Check sheet for the modelled part. Datum: model origin and axes. Units: mm. Give positions to 0.01 mm unless a question says otherwise; leave off trailing zeros. Loops run counter-clockwise (first coordinate to the right, second up) from the corner with the lowest first, then second, coordinate; pieces in that order, holes last. Notation, with made-up numbers: (15, 72.5) - (70, 72.5) arc R7 cw to (70, 81.5) - close; hole circle Ø7 at (-18, -29). An arc over 180 degrees is marked (long way). Answer in a Markdown table with one row per item. Add a question column.
(1) Draft check along Z on faces 1 (the face through (-2.44, 0.69, -0.54)), 2 (the face through (-1.22, -0.69, -0.27)). Enter one of: released by +Z, released by -Z, zero draft, split by the parting line, or undercut.
(2) Go/stop test with a flat-tipped pin: P1, Ø3, axis at x = 0, z = 0, coming from the +Y side. Record where the tip stops, or that it passes through.
(3) Sectioned sample at A-A on x = 0. Enter the section's corners in (y, z), then the cut area to 3 significant figures.
(4) Sectioned sample at B-B on z = 0. Enter the section's corners in (x, y), then the cut area to 3 significant figures.
(5) Sectioned sample at C-C on y = -22.5. Enter the section's corners in (x, z).
(6) Thickness scan on L1, parallel to X at y = -8, z = 0; L2, parallel to Y at x = -1.15, z = -1.3; L3, parallel to X at y = 38, z = 1.5. Record the ranges inside material, lowest first.
from build123d import *

# Parameters (mm, degrees)
SKETCH1_R      = 2.5
SKETCH1_R_2    = 1.25
EXTRUDE1_DEPTH = 50
CHAMFER1_SIZE  = 0.5


with BuildPart() as part:
    # Sketch1 → Extrude1 (new, symmetric)
    with BuildSketch(Plane(origin=(0, 0, 0), x_dir=(1, 0, 0), z_dir=(0, 1, 0))):
        with Locations(Location((0, 0, 0), (0, 0, 270))):
            Circle(SKETCH1_R)
        with Locations(Location((0, 0, 0), (0, 0, 270))):
            Circle(SKETCH1_R_2, mode=Mode.SUBTRACT)
    extrude(amount=EXTRUDE1_DEPTH, both=True)

    # Chamfer1
    chamfer1_edges = [part.edges().sort_by_distance(p)[0] for p in [
        (0, -50, -2.5),
        (0, 50, -2.5),
        (0, -50, -1.25),
        (0, 50, -1.25),
    ]]
    chamfer(chamfer1_edges, length=CHAMFER1_SIZE)


solid = part.part
Reply:
| question | item | result |
|---|---|---|
| 1 | face 1 | split by the parting line |
| 1 | face 2 | undercut |
| 2 | P1 | y = 49.75 |
| 3 | outline | (-50, -2) - (-49.5, -2.5) - (49.5, -2.5) - (50, -2) - (50, -1.75) - (49.5, -1.25) - (-49.5, -1.25) - (-50, -1.75) - close; (-50, 1.75) - (-49.5, 1.25) - (49.5, 1.25) - (50, 1.75) - (50, 2) - (49.5, 2.5) - (-49.5, 2.5) - (-50, 2) - close |
| 3 | area | 249 mm^2 |
| 4 | outline | (-2.5, -49.5) - (-2, -50) - (-1.75, -50) - (-1.25, -49.5) - (-1.25, 49.5) - (-1.75, 50) - (-2, 50) - (-2.5, 49.5) - close; (1.25, -49.5) - (1.75, -50) - (2, -50) - (2.5, -49.5) - (2.5, 49.5) - (2, 50) - (1.75, 50) - (1.25, 49.5) - close |
| 4 | area | 249 mm^2 |
| 5 | outline | circle Ø5 at (0, 0); hole circle Ø2.5 at (0, 0) |
| 6 | L1 | -2.5 to -1.25, 1.25 to 2.5 |
| 6 | L2 | -49.99 to 49.99 |
| 6 | L3 | -2 to 2 |
